For this review, take the finished solid that the model builds, in its own axes (mm). Give positions to 0.01 mm unless a question says otherwise; leave off trailing zeros. Loops run counter-clockwise (first coordinate to the right, second up) from the corner with the lowest first, then second, coordinate; pieces in that order, holes last. Notation, with made-up numbers: (76.5, 54.5) - (112.5, 54.5) arc R25 ccw to (112.5, 88.5) - close; hole circle Ø2 at (34, 46.25). An arc over 180 degrees is marked (long way). Answer in a Markdown table with one row per item.
```python
from build123d import *

# Parameters (mm, degrees)
F0_R     = 1.75
F1_DEPTH = 0.75
F2_SIZE  = 0.2
F3_R     = 16
F4_DEPTH = 0.2808333333
F5_SCALE = 3


with BuildPart() as f1:
    # F0 (on Top) → F1 (new body, symmetric)
    with BuildSketch(Plane.XY):
        with BuildLine():
            ThreePointArc((-1.1949222327, 13.4470130831), (0.5293090333, 15.1574275431), (2.1300276773, 13.3309032738))
            ThreePointArc((2.1300276773, 13.3309032738), (2.7028519806, 12.7159188095), (3.4762897375, 13.0447464391))
            ThreePointArc((3.4762897375, 13.0447464391), (5.6815333335, 14.0622884609), (6.5610087387, 11.7984390633))
            ThreePointArc((6.5610087387, 11.7984390633), (6.888950435, 11.02462525), (7.7282098608, 11.0690908546))
            ThreePointArc((7.7282098608, 11.0690908546), (9.6681759929, 11.5734494675), (10.6897886008, 9.8488759309))
            Line((10.6897886008, 9.8488759309), (10.6042593257, 9.0771032695))
            ThreePointArc((10.6042593257, 9.0771032695), (11.2613895868, 8.3010656426), (12, 9))
            Line((12, 9), (12, 15.8830052443))
            ThreePointArc((12, 15.8830052443), (-2.2823101594, 21.1363840676), (-14.5, 12.0638746292))
            Line((-14.5, 12.0638746292), (-14.5, 6.4923420176))
            ThreePointArc((-14.5, 6.4923420176), (-13.8076579824, 5.8), (-13.1153159648, 6.4923420176))
            Line((-13.1153159648, 6.4923420176), (-13.1153159648, 7.1539100671))
            ThreePointArc((-13.1153159648, 7.1539100671), (-12.0573735414, 8.7054359527), (-10.2266368767, 8.2872517719))
            ThreePointArc((-10.2266368767, 8.2872517719), (-10.0691213433, 8.2512714446), (-9.9780965836, 8.3847638426))
            Line((-9.9780965836, 8.3847638426), (-9.9780965836, 10.6381451737))
            ThreePointArc((-9.9780965836, 10.6381451737), (-8.8304088419, 12.2219502921), (-6.9679701997, 11.624498947))
            ThreePointArc((-6.9679701997, 11.624498947), (-6.2690751364, 11.4003005298), (-5.8383960907, 11.9946361248))
            Line((-5.8383960907, 11.9946361248), (-5.8383960907, 12.83926297))
            ThreePointArc((-5.8383960907, 12.83926297), (-4.3814979484, 14.4926760896), (-2.557866158, 13.2554638062))
            ThreePointArc((-2.557866158, 13.2554638062), (-1.8092503125, 12.8734848936), (-1.1949222327, 13.4470130831))
        make_face()
        with Locations((0, 19)):
            Circle(F0_R, mode=Mode.SUBTRACT)
    extrude(amount=F1_DEPTH, both=True)

    # F2
    f2_edges = [f1.edges().sort_by_distance(p)[0] for p in [
        (-1.75, 19, -0.75),
    ]]
    chamfer(f2_edges, length=F2_SIZE)

    # F3 (on Top) → F4 (cut, symmetric)
    with BuildSketch(Plane.XY):
        Circle(F3_R)
    extrude(amount=F4_DEPTH, both=True, mode=Mode.SUBTRACT)


with BuildPart() as f1_1:
    # F5: moved
    add(f1.part.scale(F5_SCALE))


solid = f1_1.part
```
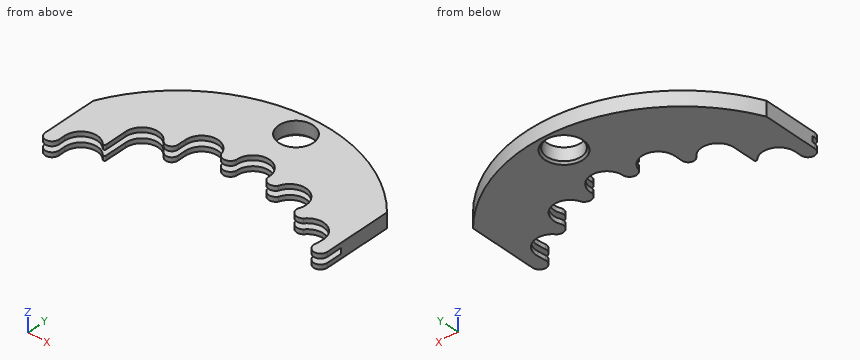
1. Wall thickness on line 1 (Y direction, x = 0, z = 0.65); line 2 (X direction, y = 36.5, z = -1.05); line 3 (X direction, y = 41, z = -1.15): over which ranges is each line inside the solid? List them lowest first. Write a range as [from, to].
Values:
| item | result |
|---|---|
| line 1 | y = [48, 51.75], [62.25, 63.9] |
| line 2 | x = [-43.35, -26.93], [-22.94, -17.52], [20.06, 36] |
| line 3 | x = [-40.91, -16.86], [-8.17, -3.56], [6.39, 11.55], [18.79, 36] |
2. Clearance check with flat-ended pins moving along their axes: pin 1 (15.5 mm diameter, centred on x = -8, y = 27.5, fed in from -Z); pin 2 (2 mm diameter, centred on x = -3.5, z = -0.5, fed in from -Y); pin 3 (1.5 mm diameter, centred on y = 20, z = 1.5, fed in from +X). State where each tip first meets the part, or that it passes through.
Values:
| item | result |
|---|---|
| pin 1 | passes through |
| pin 2 | stops at y = 39.02 |
| pin 3 | stops at x = -39.35 |
3. We need section D-D, the plane x = 8.5. Give the boundary of the cut face in (y, z).
Values:
| item | result |
|---|---|
| outline | (38.1, -2.25) - (63.14, -2.25) - (63.14, 2.25) - (38.1, 2.25) - (38.1, 0.84) - (47.24, 0.84) - (47.24, -0.84) - (38.1, -0.84) - close |
4. We need section B-B, the plane x = 0. Give the boundary of the cut face in (y, z), and give its area (3 significant figures).
Values:
| item | result |
|---|---|
| outline | (45.27, -2.25) - (51.15, -2.25) - (51.75, -1.65) - (51.75, 2.25) - (45.27, 2.25) - (45.27, 0.84) - (48, 0.84) - (48, -0.84) - (45.27, -0.84) - close; (62.25, -1.65) - (62.85, -2.25) - (63.9, -2.25) - (63.9, 2.25) - (62.25, 2.25) - close |
| area | 31.6 mm^2 |
5. We need section A-A, the plane y = 57. Give the boundary of the cut face in (x, z).
Values:
| item | result |
|---|---|
| outline | (-24.79, -2.25) - (-5.85, -2.25) - (-5.25, -1.65) - (-5.25, 2.25) - (-24.79, 2.25) - close; (5.25, -1.65) - (5.85, -2.25) - (24.79, -2.25) - (24.79, 2.25) - (5.25, 2.25) - close |
6. We need section C-C, the plane x = 30. Give the boundary of the cut face in (y, z), and give its area (3 significant figures).
Values:
| item | result |
|---|---|
| outline | (34.17, -2.25) - (53.37, -2.25) - (53.37, 2.25) - (34.17, 2.25) - (34.17, 0.84) - (37.47, 0.84) - (37.47, -0.84) - (34.17, -0.84) - close |
| area | 80.8 mm^2 |
